from build123d import *

# Parameters (mm, degrees)
SKETCH1_R           = 30
BOSS_EXTRUDE1_DEPTH = 3
SKETCH2_R           = 2
CUT_EXTRUDE1_DEPTH  = 3
SKETCH3_R           = 3
BOSS_EXTRUDE2_DEPTH = 32
FILLET1_R           = 0.5


with BuildPart() as part:
    # Sketch1 → Boss-Extrude1 (new body)
    with BuildSketch(Plane(origin=(0, 0, 0), x_dir=(0, 0, -1), z_dir=(1, 0, 0))):
        Circle(SKETCH1_R)
    extrude(amount=BOSS_EXTRUDE1_DEPTH)

    # Sketch2 → Cut-Extrude1 (cut)
    with BuildSketch(Plane(origin=(0, 0, 0), x_dir=(0, 0, -1), z_dir=(1, 0, 0))):
        with Locations((20.7, 0)):
            Circle(SKETCH2_R)
        with Locations((10.35, -17.926725858)):
            Circle(SKETCH2_R)
        with Locations((-10.35, -17.926725858)):
            Circle(SKETCH2_R)
        with Locations((-20.7, 0)):
            Circle(SKETCH2_R)
        with Locations((-10.35, 17.926725858)):
            Circle(SKETCH2_R)
        with Locations((10.35, 17.926725858)):
            Circle(SKETCH2_R)
    extrude(amount=CUT_EXTRUDE1_DEPTH, mode=Mode.SUBTRACT)

    # Sketch3 → Boss-Extrude2 (add)
    with BuildSketch(Plane(origin=(3, 0, 0), x_dir=(0, 0, -1), z_dir=(1, 0, 0))):
        Circle(SKETCH3_R)
    extrude(amount=BOSS_EXTRUDE2_DEPTH)

    # Fillet1
    fillet1_edges = [part.edges().sort_by_distance(p)[0] for p in [
        (35, 0, 3),
    ]]
    fillet(fillet1_edges, radius=FILLET1_R)


solid = part.part
Here's how the part is built. I have some questions about the finished solid (model axes, mm). Coordinates: 2 decimals unless noted, no trailing zeros. Order: outer loops, then holes, each group sorted by start corner. A loop starts at its lowest first (then second) coordinate and runs counter-clockwise, first axis right, second up. Notation, with made-up numbers: M 88,1 L 107,1 A17 cw 107,5 Z; hole C 64,84.25 d1. An arc over 180 degrees is marked long. Answer as CSV lines item,"result". Start each with the question number.
1. I want a section at D-D, the plane z = 10.35. Write out the boundary of the cut face in (x, y).
2. I want a section at B-B, the plane z = 20.5. Write out the boundary of the cut face in (x, y).
3. I want a section at A-A, the plane y = 0. Write out the boundary of the cut face in (x, z), and give its area (3 significant figures).
4. For pin 1 (5 mm diameter, centred on y = 22.5, z = -7, fed in from +X); pin 2 (12 mm diameter, centred on x = 27, z = 8.5, fed in from +Y); pin 3 (4 mm diameter, centred on x = 10, z = 2, fed in from +Y), each with a flat end and sliding along its axis, tell me the tip position at first contact or that it passes through.
5. We'd pull the mould along Z, two halves only. Please class faces 1 (the cylindrical face through (19, 0, 3)), 2 (the flat face through (0, 0, 0)), 3 (the cylindrical face through (1.479, 0.088, 22.698)): released by +Z, released by -Z, zero draft, split by the parting line, or undercut.
6. I want a section at C-C, the plane z = 0. Write out the boundary of the cut face in (x, y), and give its area (3 significant figures).
7. I need wall thicknesses on line 1 (Y direction, x = 1, z = -10); line 2 (X direction, y = -16.5, z = -15.5); line 3 (Y direction, x = 1, z = 20). Which ranges of each line are inside material? Lowest first, please. Write a range as [from, to].
Recorded:
1,outline,"M 0,-28.16 L 3,-28.16 L 3,-19.93 L 0,-19.93 Z; M 0,-15.93 L 3,-15.93 L 3,15.93 L 0,15.93 Z; M 0,19.93 L 3,19.93 L 3,28.16 L 0,28.16 Z"
2,outline,"M 0,-21.9 L 3,-21.9 L 3,-1.99 L 0,-1.99 Z; M 0,1.99 L 3,1.99 L 3,21.9 L 0,21.9 Z"
3,outline,"M 0,-30 L 3,-30 L 3,-22.7 L 0,-22.7 Z; M 0,-18.7 L 3,-18.7 L 3,-3 L 34.5,-3 A0.5 ccw 35,-2.5 L 35,2.5 A0.5 ccw 34.5,3 L 3,3 L 3,18.7 L 0,18.7 Z; M 0,22.7 L 3,22.7 L 3,30 L 0,30 Z"
3,area,"348 mm2"
4,pin 1,"stops at x = 3"
4,pin 2,"stops at y = 1.66"
4,pin 3,"stops at y = 3"
5,face 1,"split by the parting line"
5,face 2,"zero draft"
5,face 3,"undercut"
6,outline,"M 0,-30 L 3,-30 L 3,-3 L 34.5,-3 A0.5 ccw 35,-2.5 L 35,2.5 A0.5 ccw 34.5,3 L 3,3 L 3,30 L 0,30 Z"
6,area,"372 mm2"
7,line 1,"y = [-28.28, -19.9], [-15.96, 15.96], [19.9, 28.28]"
7,line 2,"x = [0, 3]"
7,line 3,"y = [-22.36, -1.87], [1.87, 22.36]"
